```python
from build123d import *

# Parameters (mm, degrees)
CROQUIS1_W              = 100
CROQUIS1_H              = 500
CROQUIS1_R              = 3.125
SALIENTE_EXTRUIR1_DEPTH = 10
CROQUIS2_W              = 150.55959244
CROQUIS2_H              = 116.869560182
SALIENTE_EXTRUIR2_DEPTH = 10


with BuildPart() as part:
    # Croquis1 → Saliente-Extruir1 (new body, symmetric)
    with BuildSketch(Plane.XY):
        Rectangle(CROQUIS1_W, CROQUIS1_H)
        with Locations((0, 150)):
            Circle(CROQUIS1_R, mode=Mode.SUBTRACT)
    extrude(amount=SALIENTE_EXTRUIR1_DEPTH, both=True)

    # Croquis2 → Saliente-Extruir2 (add, symmetric)
    with BuildSketch(Plane.XZ.offset(250)):
        Rectangle(CROQUIS2_W, CROQUIS2_H)
    extrude(amount=SALIENTE_EXTRUIR2_DEPTH, both=True)


solid = part.part
```
Source: CAD feature listing. Evaluate the final solid. Frame: model axes, mm. A direction names the side the tool comes from. Coordinates: 2 decimals unless noted, no trailing zeros. Order: outer loops, then holes, each group sorted by start corner. A loop starts at its lowest first (then second) coordinate and runs counter-clockwise, first axis right, second up. Notation, with made-up numbers: (10.5, 49.5) - (60.5, 49.5) arc R24 ccw to (60.5, 61.5) - close; hole circle Ø6 at (54, 69.25). An arc over 180 degrees is marked (long way). One line per item, written item: value.
1) Contact query for flat-ended pins moving along their axis: pin 1 (6 mm diameter, centred on x = 2.5, z = -18.5, fed in from +Y); pin 2 (22 mm diameter, centred on y = 55.5, z = 2.5, fed in from -X); pin 3 (22 mm diameter, centred on y = 9, z = 1, fed in from +X). Output: stop coordinate, or through.
Computed values:
pin 1: stops at y = -240
pin 2: stops at x = -50
pin 3: stops at x = 50
2) Cut plane D-D on y = -63.5. Output: boundary loops of the cut face in (x, z).
Computed values:
outline: (-50, -10) - (50, -10) - (50, 10) - (-50, 10) - close
3) Ray query, line 1 (X direction, y = 150, z = 4) (3 decimals); line 2 (Y direction, x = 0, z = -1) (3 decimals); line 3 (Y direction, x = -54.5, z = -36). Return the intervals inside material, ascending. Write a range as [from, to].
Computed values:
line 1: x = [-50, -3.125], [3.125, 50]
line 2: y = [-260, 146.875], [153.125, 250]
line 3: y = [-260, -240]
4) Cut plane B-B on x = -21.5. Output: boundary loops of the cut face in (y, z), plus the area to 3 significant figures.
Computed values:
outline: (-260, -58.43) - (-240, -58.43) - (-240, -10) - (250, -10) - (250, 10) - (-240, 10) - (-240, 58.43) - (-260, 58.43) - close
area: 12,100 mm^2
5) Reachability of faces 1 (the face through (-50, 2, 0)), 2 (the face through (-1, 8, -10)), 3 (the face through (-1, 8, 10)) from +Z, -Z, +X, -X, +Y, -Y: full face, straight path, thin tool, end or side. Return the list, or none.
Computed values:
face 1: +Z, -Z, -X, +Y
face 2: -Z, +X, -X, +Y
face 3: +Z, +X, -X, +Y
6) Cut plane A-A on z = -3. Output: boundary loops of the cut face in (x, y) (3 decimals).
Computed values:
outline: (-75.28, -260) - (75.28, -260) - (75.28, -240) - (50, -240) - (50, 250) - (-50, 250) - (-50, -240) - (-75.28, -240) - close; hole circle Ø6.25 at (0, 150)
7) Cut plane C-C on z = 46. Output: boundary loops of the cut face in (x, y).
Computed values:
outline: (-75.28, -260) - (75.28, -260) - (75.28, -240) - (-75.28, -240) - close
